from build123d import *

# Parameters (mm, degrees)
BOSS_EXTRUDE1_DEPTH = 3.175
MIRROR1_OUTLINE_W   = 6.35
MIRROR1_OUTLINE_H   = 3.175
MIRROR1_DEPTH       = 248.225
MIRROR1_2_OUTLINE_W = 104.175
MIRROR1_2_OUTLINE_H = 3.175
MIRROR1_2_DEPTH     = 6.35
MIRROR1_START       = 84.858333333
MIRROR1_3_OUTLINE_W = 6.35
MIRROR1_3_OUTLINE_H = 3.175
MIRROR1_3_DEPTH     = 75.333333334
MIRROR1_START_2     = 6.35
MIRROR1_4_OUTLINE_W = 30.491666667
MIRROR1_4_OUTLINE_H = 3.175
MIRROR1_4_DEPTH     = 6.35
MIRROR1_START_3     = 241.875
MIRROR1_5_OUTLINE_W = 6.35
MIRROR1_5_OUTLINE_H = 3.175
MIRROR1_5_DEPTH     = 6.35
MIRROR1_START_4     = 238.7
MIRROR1_6_OUTLINE_W = 2.116666666
MIRROR1_6_OUTLINE_H = 3.175
MIRROR1_6_DEPTH     = 3.175
SKETCH2_W           = 3.175
SKETCH2_H           = 3.175
CUT_EXTRUDE1_DEPTH  = 3.175


# Read off the part's stored shape, not the designer's step: Mirror1
with BuildPart() as part:
    # Sketch1 → Boss-Extrude1 (new body)
    with BuildSketch(Plane.XY):
        Polygon((6.35, 232.35), (0, 232.35), (0, 0), (110.525, 0), (110.525, 12.7), (80.033333333, 12.7), (80.033333333, 6.35), (6.35, 6.35), (6.35, 84.858333333), (12.7, 84.858333333), (12.7, 160.191666667), (6.35, 160.191666667), align=None)
        Polygon((-2.116666667, 241.875), (0, 241.875), (0, 232.35), (6.35, 232.35), (6.35, 248.225), (-6.35, 248.225), (-6.35, 241.875), (-4.233333333, 241.875), (-4.233333333, 238.7), (-2.116666667, 238.7), align=None)
    extrude(amount=BOSS_EXTRUDE1_DEPTH)



with BuildPart() as body_2:
    # Mirror1 outline → Mirror1 (new body)
    with BuildSketch(Plane(origin=(0, 0, 0), x_dir=(1, 0, 0), z_dir=(0, 1, 0))):
        with Locations((217.875, -1.5875)):
            Rectangle(MIRROR1_OUTLINE_W, MIRROR1_OUTLINE_H)
    extrude(amount=MIRROR1_DEPTH)


with BuildPart() as part_1:
    add(part.part)

    add(body_2.part)  # Mirror1 2 merges body 2
    # Mirror1 2 outline → Mirror1 2 (add)
    with BuildSketch(Plane(origin=(0, 0, 0), x_dir=(1, 0, 0), z_dir=(0, 1, 0))):
        with Locations((162.6125, -1.5875)):
            Rectangle(MIRROR1_2_OUTLINE_W, MIRROR1_2_OUTLINE_H)
    extrude(amount=MIRROR1_2_DEPTH)

    # Mirror1 3 outline → Mirror1 3 (add)
    with BuildSketch(Plane(origin=(0, 0, 0), x_dir=(1, 0, 0), z_dir=(0, 1, 0)).offset(MIRROR1_START)):
        with Locations((211.525, -1.5875)):
            Rectangle(MIRROR1_3_OUTLINE_W, MIRROR1_3_OUTLINE_H)
    extrude(amount=MIRROR1_3_DEPTH)

    # Mirror1 4 outline → Mirror1 4 (add)
    with BuildSketch(Plane(origin=(0, 0, 0), x_dir=(1, 0, 0), z_dir=(0, 1, 0)).offset(MIRROR1_START_2)):
        with Locations((125.770833334, -1.5875)):
            Rectangle(MIRROR1_4_OUTLINE_W, MIRROR1_4_OUTLINE_H)
    extrude(amount=MIRROR1_4_DEPTH)

    # Mirror1 5 outline → Mirror1 5 (add)
    with BuildSketch(Plane(origin=(0, 0, 0), x_dir=(1, 0, 0), z_dir=(0, 1, 0)).offset(MIRROR1_START_3)):
        with Locations((224.225, -1.5875)):
            Rectangle(MIRROR1_5_OUTLINE_W, MIRROR1_5_OUTLINE_H)
    extrude(amount=MIRROR1_5_DEPTH)

    # Mirror1 6 outline → Mirror1 6 (add)
    with BuildSketch(Plane(origin=(0, 0, 0), x_dir=(1, 0, 0), z_dir=(0, 1, 0)).offset(MIRROR1_START_4)):
        with Locations((224.225, -1.5875)):
            Rectangle(MIRROR1_6_OUTLINE_W, MIRROR1_6_OUTLINE_H)
    extrude(amount=MIRROR1_6_DEPTH)

    # Sketch2 → Cut-Extrude1 (cut)
    with BuildSketch(Plane.XY.offset(3.175)):
        with Locations((75.270833333, 1.5875)):
            Rectangle(SKETCH2_W, SKETCH2_H)
        with Locations((145.779166667, 4.7625)):
            Rectangle(SKETCH2_W, SKETCH2_H)
    extrude(amount=-CUT_EXTRUDE1_DEPTH, mode=Mode.SUBTRACT)


solid = part_1.part
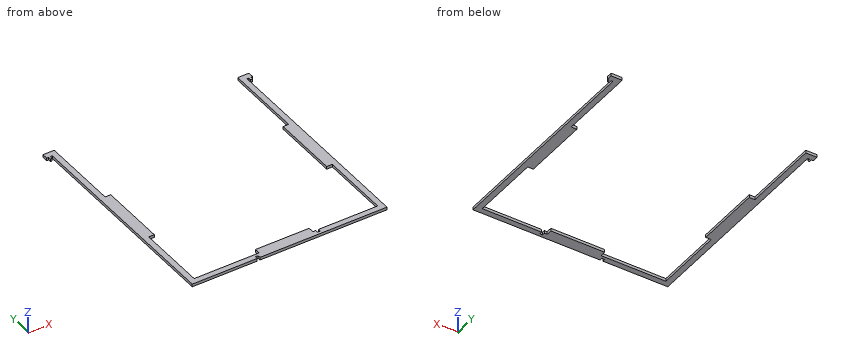
Can you work these out from the model? Positions are in its coordinate system, mm. Coordinates: 2 decimals unless noted, no trailing zeros. Loops run counter-clockwise (first coordinate to the right, second up) from the corner with the lowest first, then second, coordinate; pieces in that order, holes last. Notation, with made-up numbers: (55, -6) - (106, -6) arc R21 ccw to (106, -2) - close; hole circle Ø2 at (-4, 72.25). An arc over 180 degrees is marked (long way). Answer as a JSON object with one key per item and string values. Group by question number.
Item 1: If we section it at D-D (x = 135): List the corners of the cut face in (y, z) for me (3 decimals), plus the area to 3 significant figures.
Item 2: If I drill on L1, parallel to X at y = 102, z = 0.5; L2, parallel to X at y = 33, z = 2.25; L3, parallel to Y at x = 211, z = 1.05, over which ranges is the centre line in solid material (lowest first)? Write a range as from..to.
Item 3: For pin 1 (1.6 mm diameter, centred on y = 111.5, z = 1.5, fed in from -X); pin 2 (1.7 mm diameter, centred on x = 224.5, z = 1.5, fed in from -Y); pin 3 (1.6 mm diameter, centred on x = 112.5, z = 1.5, fed in from +Y), each with a flat end and sliding along its axis, tell me the tip position at first contact or that it passes through.
Item 4: If we section it at A-A (y = 120): List the corners of the cut face in (x, z) for me (3 decimals), plus the area to 3 significant figures.
Item 5: If we section it at B-B (x = 176): List the corners of the cut face in (y, z) for me (3 decimals), plus the area to 3 significant figures.
Item 6: If we section it at C-C (y = 174.5): List the corners of the cut face in (x, z) for me (3 decimals).
Returned:
{
 "1": {"outline": "(0, 0) - (12.7, 0) - (12.7, 3.175) - (0, 3.175) - close", "area": "40.3 mm²"},
 "2": {"L1": "x = 0..12.7, 208.35..221.05", "L2": "x = 0..6.35, 214.7..221.05", "L3": "y = 0..6.35, 84.86..160.19"},
 "3": {"pin 1": "stops at x = 0", "pin 2": "stops at y = 238.7", "pin 3": "stops at y = 12.7"},
 "4": {"outline": "(0, 0) - (12.7, 0) - (12.7, 3.175) - (0, 3.175) - close; (208.35, 0) - (221.05, 0) - (221.05, 3.175) - (208.35, 3.175) - close", "area": "80.6 mm²"},
 "5": {"outline": "(0, 0) - (6.35, 0) - (6.35, 3.175) - (0, 3.175) - close", "area": "20.2 mm²"},
 "6": {"outline": "(0, 0) - (6.35, 0) - (6.35, 3.175) - (0, 3.175) - close; (214.7, 0) - (221.05, 0) - (221.05, 3.175) - (214.7, 3.175) - close"}
}
